Verification items for the finished model (mm, model axes). A direction names the side the tool comes from. Give positions to 0.01 mm unless a question says otherwise; leave off trailing zeros. Order: outer loops, then holes, each group sorted by start corner. A loop starts at its lowest first (then second) coordinate and runs counter-clockwise, first axis right, second up.
from build123d import *

# Parameters (mm, degrees)
F0_W      = 60
F0_H      = 10
F1_DEPTH  = 40
F2_R      = 7.5
F3_DEPTH  = 10
F4_R      = 7.5
F5_DEPTH  = 10
F6_R      = 17
F7_DEPTH  = 3
F8_R      = 10
F9_DEPTH  = 25
F11_DEPTH = 10


with BuildPart() as f1:
    # F0 (on Front) → F1 (new body)
    with BuildSketch(Plane.XZ):
        with Locations((0, -0.633379)):
            Rectangle(F0_W, F0_H)
    extrude(amount=-F1_DEPTH)

    # F2 (on face) → F3 (join)
    with BuildSketch(Plane.YZ.offset(30)):
        with BuildLine():
            Line((5, 26.366621), (5, 4.366621))
            Line((5, 4.366621), (35, 4.366621))
            Line((35, 4.366621), (35, 26.366621))
            ThreePointArc((35, 26.366621), (20, 41.366621), (5, 26.366621))
        make_face()
        with Locations((20, 26.366621)):
            Circle(F2_R, mode=Mode.SUBTRACT)
    extrude(amount=-F3_DEPTH)

    # F4 (on face) → F5 (join)
    with BuildSketch(Plane(origin=(-30, 0, 0), x_dir=(0, -1, 0), z_dir=(-1, 0, 0))):
        with BuildLine():
            Line((-35, 4.366621), (-5, 4.366621))
            Line((-5, 4.366621), (-5, 26.366621))
            ThreePointArc((-5, 26.366621), (-20, 41.366621), (-35, 26.366621))
            Line((-35, 26.366621), (-35, 4.366621))
        make_face()
        with Locations((-20, 26.366621)):
            Circle(F4_R, mode=Mode.SUBTRACT)
    extrude(amount=-F5_DEPTH)

    # F6 (on face) → F7 (join)
    with BuildSketch(Plane(origin=(0, 0, -5.633379), x_dir=(1, 0, 0), z_dir=(0, 0, -1))):
        with Locations((0, -20)):
            Circle(F6_R)
    extrude(amount=F7_DEPTH)

    # F8 (on face) → F9 (cut)
    with BuildSketch(Plane.XY.offset(4.366621)):
        with Locations((0, 20)):
            Circle(F8_R)
    extrude(amount=-F9_DEPTH, mode=Mode.SUBTRACT)

    # F10 (on face) → F11 (join)
    with BuildSketch(Plane.XY.offset(4.366621)):
        with BuildLine():
            Line((17.320508, 0), (-17.320508, 0))
            ThreePointArc((-17.320508, 0), (0, -10), (17.320508, 0))
        make_face()
        with BuildLine():
            Line((-17.320508, 40), (17.320508, 40))
            ThreePointArc((17.320508, 40), (0, 50), (-17.320508, 40))
        make_face()
    extrude(amount=-F11_DEPTH)


solid = f1.part
(1) Scan lines: line 1 (Z direction, x = 27.5, y = 20); line 2 (X direction, y = 7, z = 20.5); line 3 (X direction, y = 14, z = 0.5). Record each from-to range of solid material in increasing order.
Solved:
line 1: z = -5.63 to 18.87, 33.87 to 41.37
line 2: x = -30 to -20, 20 to 30
line 3: x = -30 to -8, 8 to 30
(2) Section check A-A, the plane z = 14.5. Enter the section's corners in (x, y).
Solved:
outline: (-30, 5) - (-20, 5) - (-20, 35) - (-30, 35) - close; (20, 5) - (30, 5) - (30, 35) - (20, 35) - close
(3) Section check C-C, the plane y = 20. Enter the section's corners in (x, z).
Solved:
outline: (-30, -5.63) - (-17, -5.63) - (-17, -8.63) - (-10, -8.63) - (-10, 4.37) - (-20, 4.37) - (-20, 18.87) - (-30, 18.87) - close; (-30, 33.87) - (-20, 33.87) - (-20, 41.37) - (-30, 41.37) - close; (10, -8.63) - (17, -8.63) - (17, -5.63) - (30, -5.63) - (30, 18.87) - (20, 18.87) - (20, 4.37) - (10, 4.37) - close; (20, 33.87) - (30, 33.87) - (30, 41.37) - (20, 41.37) - close
(4) Release check for a two-part mould opening along Y. For faces 1 (the flat face through (25, 5, 16)), 2 (the flat face through (20, 16, 19)), 3 (the cylindrical face through (25.07, 14.05, 21.8)) record: pulls with the +Y half, pulls with the -Y half, needs draft (parallel to the pull), parting line crosses it, or undercut.
Solved:
face 1: pulls with the -Y half
face 2: needs draft
face 3: undercut
(5) Section check B-B, the plane x = 0. Enter the section's corners in (y, z), then the cut area to 3 significant figures.
Solved:
outline: (-10, -5.63) - (3, -5.63) - (3, -8.63) - (10, -8.63) - (10, 4.37) - (-10, 4.37) - close; (30, -8.63) - (37, -8.63) - (37, -5.63) - (50, -5.63) - (50, 4.37) - (30, 4.37) - close
area: 442 mm2
(6) Go/stop test with flat-tipped pins: pin 1 (12 mm diameter, centred on x = -23, z = 15.5, fed in from +Y); pin 2 (11 mm diameter, centred on x = 21, z = 1, fed in from +Y); pin 3 (5 mm diameter, centred on x = -21.5, z = -1, fed in from -Y). Record where each tip stops, or that it passes through.
Solved:
pin 1: stops at y = 35
pin 2: stops at y = 42.64
pin 3: stops at y = 0
(7) Set-up check for faces 4 (the flat face through (24, 0, -1)), 5 (the flat face through (24, 40, -1)), 6 (the flat face through (-14, 33, -5.633)), 7 (the flat face through (-24, 40, -1)): record each of +Z, -Z, +X, -X, +Y, -Y from which the full face is reachable in a straight line by a thin tool's end or side.
Solved:
face 4: +Z, -Z, +X, -Y
face 5: +Z, -Z, +X, +Y
face 6: -Z
face 7: +Z, -Z, -X, +Y
(8) Section check D-D, the plane x = 21. Enter the section's corners in (y, z).
Solved:
outline: (0, -5.63) - (40, -5.63) - (40, 4.37) - (35, 4.37) - (35, 26.37) arc R15 ccw to (5, 26.37) - (5, 4.37) - (0, 4.37) - close; hole circle Ø15 at (20, 26.37)
